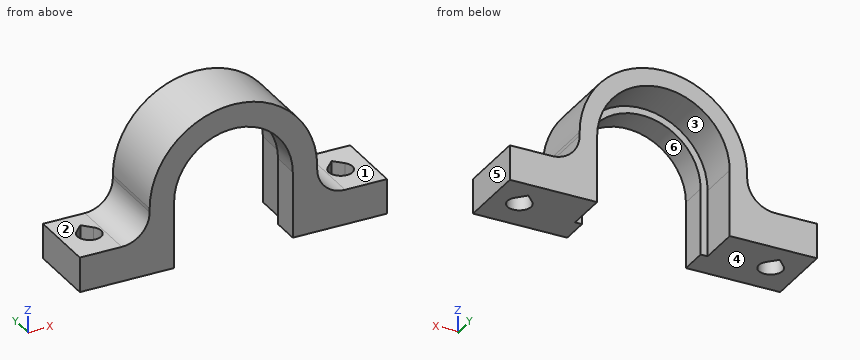
Solid Edge part; units mm, degrees
sketch "Sketch1" plane through (0, 0, 0) normal (0, -1, 0) x (1, 0, 0)
  line L0 (22, 0) -> (22, 5)
  line L1 (22, 5) -> (16, 5)
  arc A0 (12, 9) -> (16, 5) centre (16, 9) ccw
  line L2 (12, 9.5) -> (12, 9)
  line L3 (-12, 9.5) -> (-12, 9)
  arc A1 (-16, 5) -> (-12, 9) centre (-16, 9) ccw
  line L4 (-16, 5) -> (-22, 5)
  line L5 (-22, 5) -> (-22, 0)
  line L6 (-22, 0) -> (-9.5, 0)
  line L7 (-9.5, 9.5) -> (-9.5, 0)
  line L8 (9.5, 9.5) -> (9.5, 0)
  line L9 (9.5, 0) -> (22, 0)
  arc A2 (12, 9.5) -> (-12, 9.5) centre (0, 9.5) ccw
  arc A3 (-9.5, 9.5) -> (9.5, 9.5) centre (0, 9.5) cw
  dimension "D1" = 22
extrude "Protrusion1" add sketch "Sketch1" along normal blind 10
sketch "Sketch2" plane through (10.6847, -6, 5) normal (0, 0, 1) x (1, 0, 0)
  line L0 (-29.9125, 2.1758) -> (-28.6898, 3.4526)
  line L1 (-28.6898, 3.4526) -> (-27.4618, 2.1809)
  arc A0 (-29.9125, 2.1758) -> (-27.4618, 2.1809) centre (-28.6847, 1) ccw
extrude "Cutout1" cut sketch "Sketch2" against normal through all
mirror "Mirror1" about plane through (0, 0, 0) normal (1, 0, 0) of "Cutout1"
sketch "Sketch3" plane through (0, -10, 10.75) normal (0, -1, 0) x (1, 0, 0)
  line L0 (-9.5, -10.75) -> (-9.5, -1.25)
  line L1 (9.5, -1.25) -> (9.5, -10.75)
  line L2 (8.5, -10.75) -> (9.5, -10.75)
  line L3 (8.5, -1.25) -> (8.5, -10.75)
  arc A0 (-8.5, -1.25) -> (8.5, -1.25) centre (0, -1.25) cw
  line L4 (-8.5, -10.75) -> (-8.5, -1.25)
  line L5 (-8.5, -10.75) -> (-9.5, -10.75)
  arc A1 (-9.5, -1.25) -> (9.5, -1.25) centre (0, -1.25) cw
extrude "ExtrudedProtrusion_2" add sketch "Sketch3" against normal blind 4
CAD build for the part. Positions are in the model's coordinates, mm. Face numbers are marked on the shaded views. A direction names the side the tool comes from. Coordinates: 2 decimals unless noted, no trailing zeros. Order: outer loops, then holes, each group sorted by start corner. A loop starts at its lowest first (then second) coordinate and runs counter-clockwise, first axis right, second up. Notation, with made-up numbers: (80, 51.5) -> (108, 51.5) arc R24 ccw to (108, 65.5) -> close; hole circle Ø9 at (65.5, 80). An arc over 180 degrees is marked (long way). Answer in a Markdown table with one row per item.
1) Flat gauge pins, fed straight in: P1, Ø9.5, axis at x = 2, z = 13.5, coming from the +Y side; P2, Ø0.6, axis at y = -7, z = 9.5, coming from the +X side; P3, Ø3, axis at x = 3.5, y = -6.5, coming from the -Z side. Where does each tip first touch, or does it go through?
Check values:
| item | result |
|---|---|
| P1 | y = -6 |
| P2 | x = 12 |
| P3 | z = 16.37 |
2) Band-saw the part on B-B (y = -4.5). List the corners of the cut face in (x, z), and give its area (3 significant figures).
Check values:
| item | result |
|---|---|
| outline | (-22, 0) -> (-19.62, 0) -> (-19.62, 5) -> (-22, 5) -> close; (-16.38, 0) -> (-9.5, 0) -> (-9.5, 9.5) arc R9.5 cw to (9.5, 9.5) -> (9.5, 0) -> (16.38, 0) -> (16.38, 5) -> (16, 5) arc R4 cw to (12, 9) -> (12, 9.5) arc R12 ccw to (-12, 9.5) -> (-12, 9) arc R4 cw to (-16, 5) -> (-16.38, 5) -> close; (19.62, 0) -> (22, 0) -> (22, 5) -> (19.62, 5) -> close |
| area | 206 mm2 |
3) Mould opens along X. For the marked faces 4, 5 and 6 say: pulls with the +X half, pulls with the -X half, needs draft (parallel to the pull), parting line crosses it, or undercut.
Check values:
| item | result |
|---|---|
| face 4 | needs draft |
| face 5 | pulls with the +X half |
| face 6 | undercut |
4) Band-saw the part on D-D (x = 0). List the corners of the cut face in (y, z).
Check values:
| item | result |
|---|---|
| outline | (-10, 18) -> (-6, 18) -> (-6, 19) -> (0, 19) -> (0, 21.5) -> (-10, 21.5) -> close |
5) Which spindle directions (+Z, -Z, +X, -X, +Y, -Y) get a long thin tool onto all of the face, cutting with end or side? Do the marked faces 1, 2 and 3. Say none if no direction does.
Check values:
| item | result |
|---|---|
| face 1 | +Z, +X, +Y, -Y |
| face 2 | +Z, -X, +Y, -Y |
| face 3 | -Z, +Y |
6) Band-saw the part on C-C (z = 6.75). List the corners of the cut face in (x, y).
Check values:
| item | result |
|---|---|
| outline | (-12.69, -10) -> (-8.5, -10) -> (-8.5, -6) -> (-9.5, -6) -> (-9.5, 0) -> (-12.69, 0) -> close; (8.5, -10) -> (12.69, -10) -> (12.69, 0) -> (9.5, 0) -> (9.5, -6) -> (8.5, -6) -> close |
7) Drill centre lines: line 1 (X direction, y = -5, z = 3.5); line 2 (X direction, y = -3.25, z = 9.5); line 3 (X direction, y = -8, z = 9.25). Where is each one in solid material? Low to high.
Check values:
| item | result |
|---|---|
| line 1 | -22 to -19.7, -16.3 to -9.5, 9.5 to 16.3, 19.7 to 22 |
| line 2 | -12 to -9.5, 9.5 to 12 |
| line 3 | -12 to -8.5, 8.5 to 12 |
8) Band-saw the part on A-A (z = 3.25). List the corners of the cut face in (x, y), and give its area (3 significant figures).
Check values:
| item | result |
|---|---|
| outline | (-22, -10) -> (-8.5, -10) -> (-8.5, -6) -> (-9.5, -6) -> (-9.5, 0) -> (-22, 0) -> close; (8.5, -10) -> (22, -10) -> (22, 0) -> (9.5, 0) -> (9.5, -6) -> (8.5, -6) -> close; hole (-19.23, -3.82) arc R1.7 ccw (long way) to (-16.78, -3.82) -> (-18.01, -2.55) -> close; hole (16.78, -3.82) arc R1.7 ccw (long way) to (19.23, -3.82) -> (18.01, -2.55) -> close |
| area | 238 mm2 |
